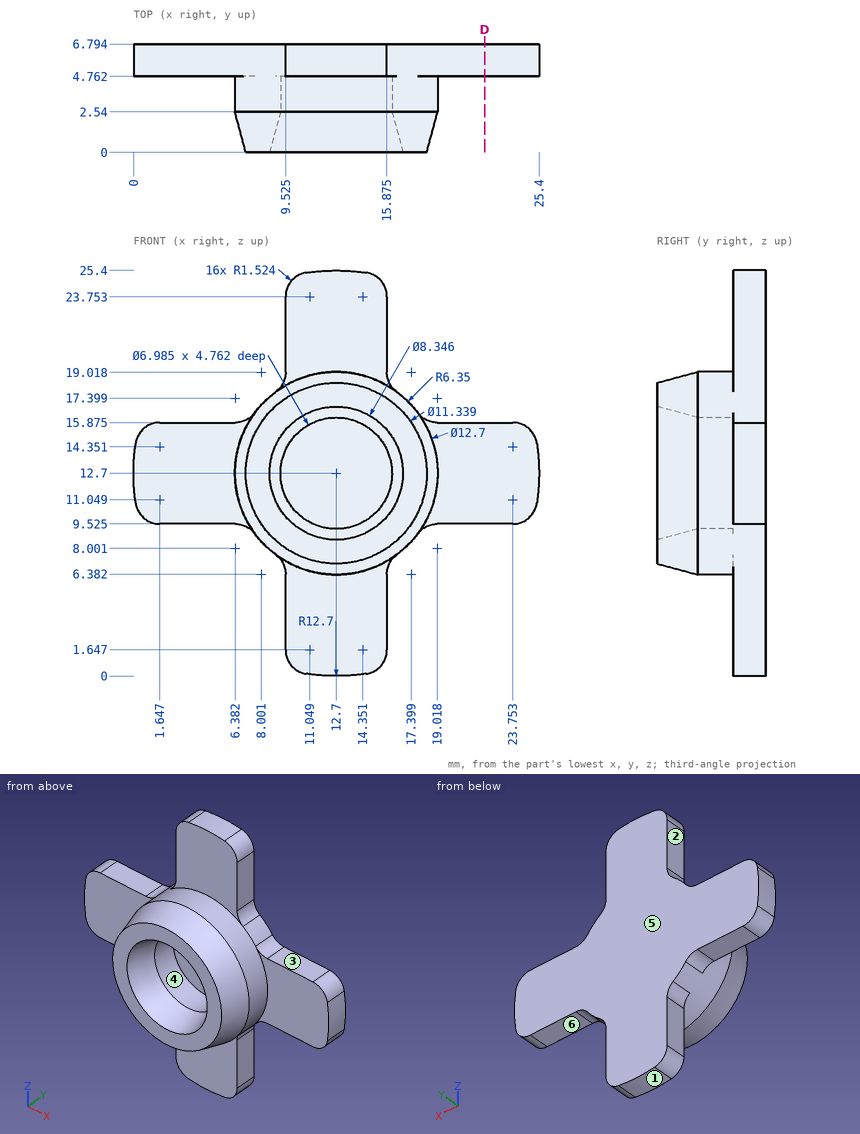
For this review, use the dimensioned drawing (mm, ordinates from the lowest corner) and the shaded views. A direction names the side the tool comes from. Give positions to 0.01 mm unless a question says otherwise; leave off trailing zeros. Order: outer loops, then holes, each group sorted by start corner. A loop starts at its lowest first (then second) coordinate and runs counter-clockwise, first axis right, second up. Notation, with made-up numbers: M 63,-33 L 76,-33 A29 ccw 76,5 Z; hole C 4,74.25 d10. An arc over 180 degrees is marked long. Use one line per item in the form item = value. Start each with the question number.
Item 1: The part is to be moulded in two halves that separate along Z. For the marked faces 4, 5 and 6, say which applies: pulls with the +Z half, pulls with the -Z half, needs draft (parallel to the pull), parting line crosses it, or undercut.
Item 2: We need section D-D on x = 22. Give the boundary of the cut face in (y, z) (1 decimal), plus the area to 3 significant figures.
Item 3: Insertion check: pin 1 Ø0.6 at (x, y) = (20.5, 5.5) entering from +Z (1 decimal); pin 2 Ø4 at (x, z) = (22.5, 13.5) entering from -Y; pin 3 Ø1 at (y, z) = (6, 3) entering from +X (1 decimal). Each pin has a flat end and moves straight along its axis. Give the tip position at first contact, or say it passes through.
Item 4: To check wall thickness, follow line 1 along X through (y, z) = (3.95, 12.7); line 2 along X through (y, z) = (5.5, 4.5) (1 decimal); line 3 along Y through (x, z) = (23, 14) (1 decimal). State the ranges of each line that lie inside material, in increasing order. Write a range as from..to.
Item 5: For the marked faces 1, 2 and 3, list the 3-axis set-ups (+Z, -Z, +X, -X, +Y, -Y) from which the entire face can be reached by the end or side of a thin tool; tool diameter is ignored.
Completed:
q1.face_4 = undercut
q1.face_5 = needs draft
q1.face_6 = pulls with the -Z half
q2.outline = M 4.8,9.5 L 6.8,9.5 L 6.8,15.9 L 4.8,15.9 Z
q2.area = 12.9 mm²
q3.pin_1 = 15.9
q3.pin_2 = 4.76
q3.pin_3 = 15.9
q4.line_1 = 6.35..9.21, 16.19..19.05
q4.line_2 = 9.5..15.9
q4.line_3 = 4.8..6.8
q5.face_1 = -Z, +Y, -Y
q5.face_2 = +Z, -X, +Y, -Y
q5.face_3 = +Z, +X, +Y, -Y
